Could you check a few things on this drawing? It's one solid part, dimensions in mm from its lowest x, y, z. A direction names the side the tool comes from. Coordinates: 2 decimals unless noted, no trailing zeros. Write each loop counter-clockwise with the first axis right and the second up, starting at its lowest first coordinate (ties: lowest second). Pieces come first, ordered by that corner, then holes. Notation, with made-up numbers: M -12,75.25 L 24,75.25 A23 ccw 24,92.25 Z; hole C 66.25,62 d9. An arc over 180 degrees is marked long. Use a Markdown table: item, result.
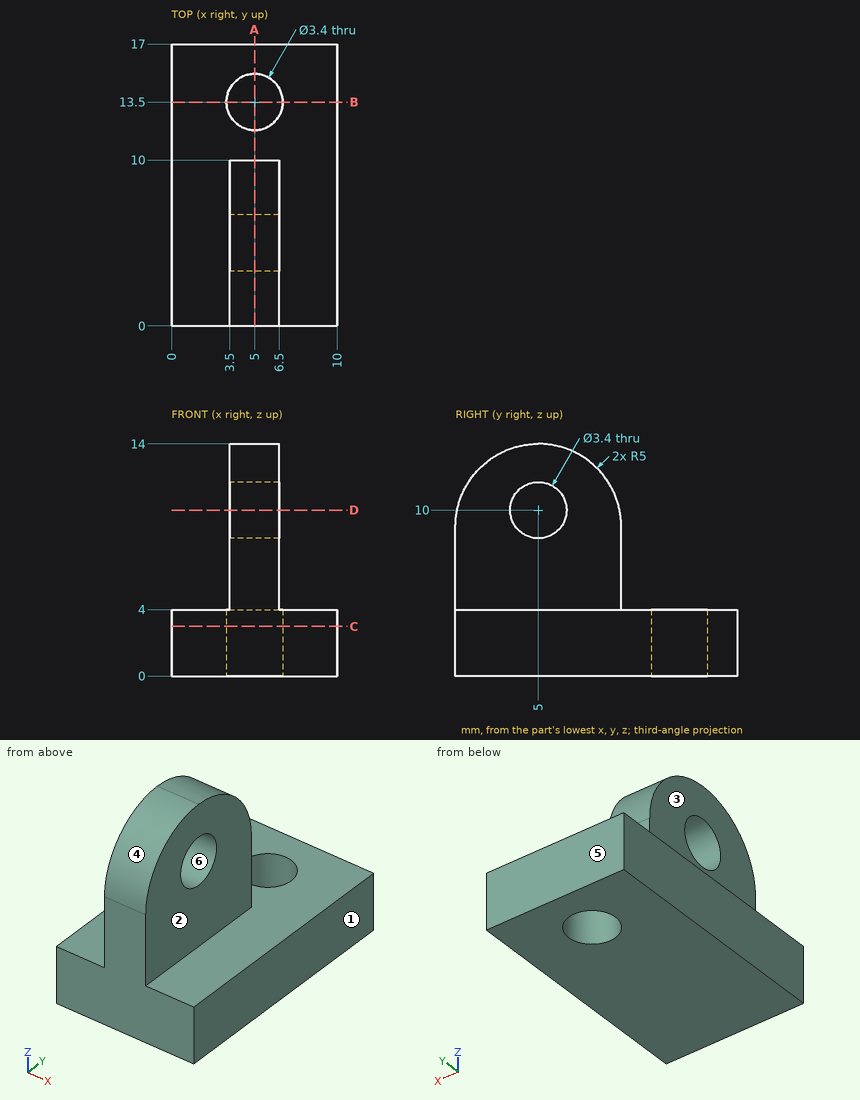
1. Will these pins go through, and if not, where does the flat tip stop? pin 1 Ø3 at (y, z) = (7.5, 8.5) entering from +X; pin 2 Ø0.9 at (x, z) = (5, 7) entering from +Y; pin 3 Ø4.5 at (x, y) = (5, 13.5) entering from +Z.
Answers follow:
| item | result |
|---|---|
| pin 1 | stops at x = 6.5 |
| pin 2 | stops at y = 10 |
| pin 3 | stops at z = 4 |
2. Suppose I cut it at D-D on z = 10. Write out the boundary of the cut face in (x, y), and give its area (3 significant figures).
Answers follow:
| item | result |
|---|---|
| outline | M 3.5,0.1 L 6.5,0.1 L 6.5,3.3 L 3.5,3.3 Z; M 3.5,6.7 L 6.5,6.7 L 6.5,9.9 L 3.5,9.9 Z |
| area | 19.2 mm2 |
3. Which directions (+Z, -Z, +X, -X, +Y, -Y) give clear straight access to the entire face, cutting with the end or side of a thin tool? Please do the marked faces 1, 2 and 3.
Answers follow:
| item | result |
|---|---|
| face 1 | +Z, -Z, +X, +Y, -Y |
| face 2 | +Z, +X, +Y, -Y |
| face 3 | +Z, -X, +Y, -Y |
4. Suppose I cut it at B-B on y = 13.5. Write out the boundary of the cut face in (x, z).
Answers follow:
| item | result |
|---|---|
| outline | M 0,0 L 3.3,0 L 3.3,4 L 0,4 Z; M 6.7,0 L 10,0 L 10,4 L 6.7,4 Z |
5. I need wall thicknesses on probe 1 along X at (y, z) = (13.5, 2.25); probe 2 along Y at (x, z) = (5, 2.2); probe 3 along X at (y, z) = (5.25, 4.75). Which ranges of each line are inside material? Lowest first, please.
Answers follow:
| item | result |
|---|---|
| probe 1 | x = 0 to 3.3, 6.7 to 10 |
| probe 2 | y = 0 to 11.8, 15.2 to 17 |
| probe 3 | x = 3.5 to 6.5 |
6. We'd pull the mould along Z, two halves only. Please class the marked faces 4, 5 and 6: +Z half, -Z half, draft (parallel to the pull), parting line (faces both ways), or undercut.
Answers follow:
| item | result |
|---|---|
| face 4 | +Z half |
| face 5 | draft |
| face 6 | undercut |
7. Suppose I cut it at A-A on x = 5. State how many separate pieces and enclosed holes the cut face has, and give its area (3 significant figures).
Answers follow:
| item | result |
|---|---|
| separate pieces | 2 |
| enclosed holes | 1 |
| area | 135 mm2 |
8. Suppose I cut it at C-C on z = 3. Write out the boundary of the cut face in (x, y), and give its area (3 significant figures).
Answers follow:
| item | result |
|---|---|
| outline | M 0,0 L 10,0 L 10,17 L 0,17 Z; hole C 5,13.5 d3.4 |
| area | 161 mm2 |
